```python
from build123d import *

# Parameters (mm, degrees)
F1_DEPTH = 25


with BuildPart() as f1:
    # F0 (on Front) → F1 (new body)
    with BuildSketch(Plane.XZ):
        Polygon((0, 0), (-25, 25), (-25, -25), (25, -25), align=None)
        Polygon((0, 25), (-25, 25), (0, 0), align=None)
    extrude(amount=-F1_DEPTH)


solid = f1.part
```
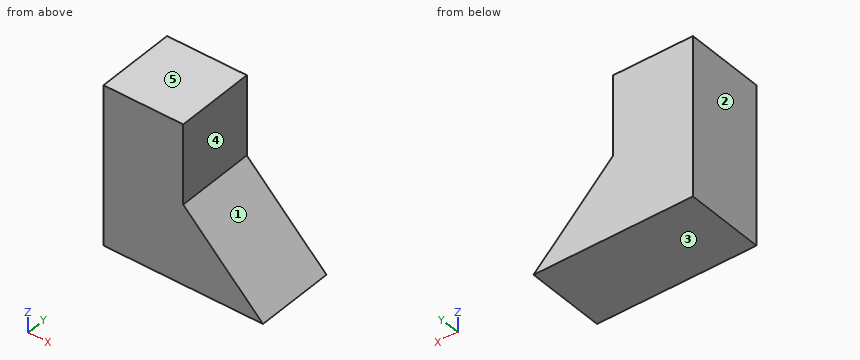
The listing builds one solid part. Answer for the finished solid, in the listing's coordinates (mm). Face numbers are marked on the shaded views. A direction names the side the tool comes from. Give positions to 0.01 mm unless a question says otherwise; leave off trailing zeros. Order: outer loops, then holes, each group sorted by start corner. A loop starts at its lowest first (then second) coordinate and runs counter-clockwise, first axis right, second up. Notation, with made-up numbers: (20, 43.25) - (72, 43.25) arc R31 ccw to (72, 77.25) - close; hole circle Ø4 at (-10.75, 67). An arc over 180 degrees is marked (long way). Use one line per item in the form item = value. Start each with the question number.
(1) Flat-ended cylindrical pins translate along their axes: pin 1 Ø6 at (x, y) = (8.5, 8) entering from +Z; pin 2 Ø12 at (x, z) = (17.5, -2.5) entering from +Y; pin 3 Ø2 at (y, z) = (9.5, -9.5) entering from +X. Find the tip coordinate at first contact, or state that the pin passes through.
(2) A cutting plane is placed at B-B, the plane x = 3.5. Write down the section's boundary in (y, z).
(3) A cutting plane is placed at C-C, the plane z = -8.5. Write down the section's boundary in (x, y).
(4) For the marked faces 4 and 5, determine the directions among +Z, -Z, +X, -X, +Y, -Y from which every point of the face is accessible in a straight line to the end or side of a thin tool.
(5) The mould has two halves that part along Z. Classify the marked faces 1, 2 and 3: released by +Z, released by -Z, zero draft, split by the parting line, or undercut.
(6) A cutting plane is placed at A-A, the plane y = 20.5. Write down the section's boundary in (x, z).
(7) Consider line 1 (X direction, y = 23.5, z = 5); line 2 (X direction, y = 14, z = -20); line 3 (Z direction, x = 17.5, y = 1.5). Determine where each line is inside the solid, lowest interval first. Write a range as from..to.
Ans:
q1.pin_1 = -5.5
q1.pin_2 = through
q1.pin_3 = 10.5
q2.outline = (0, -25) - (25, -25) - (25, -3.5) - (0, -3.5) - close
q3.outline = (-25, 0) - (8.5, 0) - (8.5, 25) - (-25, 25) - close
q4.face_4 = +Z, +X, +Y, -Y
q4.face_5 = +Z, +X, -X, +Y, -Y
q5.face_1 = released by +Z
q5.face_2 = zero draft
q5.face_3 = released by -Z
q6.outline = (-25, -25) - (25, -25) - (0, 0) - (0, 25) - (-25, 25) - close
q7.line_1 = -25..0
q7.line_2 = -25..20
q7.line_3 = -25..-17.5
